For this review, take the finished solid that the model builds, in its own axes (mm). Face numbers are marked on the shaded views. A direction names the side the tool comes from. Give positions to 0.01 mm unless a question says otherwise; leave off trailing zeros. Loops run counter-clockwise (first coordinate to the right, second up) from the corner with the lowest first, then second, coordinate; pieces in that order, holes last. Notation, with made-up numbers: (40, 59.25) - (70, 59.25) arc R31 ccw to (70, 93.25) - close; hole circle Ø10 at (77.5, -6.5). An arc over 180 degrees is marked (long way). Use CSV: the item, a comma, the result in double quotes. Start each with the question number.
1. Take a section at B-B on z = 17.5. Give the boundary of the cut face in (x, y).
2. Wall thickness on line 1 (X direction, y = -42, z = 8.5); line 2 (X direction, y = 23.5, z = 22.5); line 3 (X direction, y = 40, z = -0.5): over which ranges is each line inside the solid? List them lowest first.
3. Take a section at C-C on y = -20.5. Give the boundary of the cut face in (x, z).
4. For the marked faces 1 and 2, list the 3-axis set-ups (+Z, -Z, +X, -X, +Y, -Y) from which the entire face can be reached by the end or side of a thin tool; tool diameter is ignored.
5. For pin 1 (5.5 mm diameter, centred on x = 12.96, y = -44.14, fed in from +Z); pin 2 (10 mm diameter, centred on x = -29.54, y = 5.21, fed in from +Z); pin 3 (7 mm diameter, centred on x = 77.94, y = -43.87, fed in from -Z); pin 4 (5 mm diameter, centred on y = 69.5, z = -5, fed in from +X), all flat-tipped, find the tip position at first contact; note any pin that passes through.
6. Take a section at A-A on y = 30. Give the boundary of the cut face in (x, z), plus the area to 3 significant figures.
7. Mouldability with a two-part tool opening along Y and no side actions: class the marked faces 3, 4 and 5 as pulls with the +Y half, pulls with the -Y half, needs draft (parallel to the pull), parting line crosses it, or undercut.
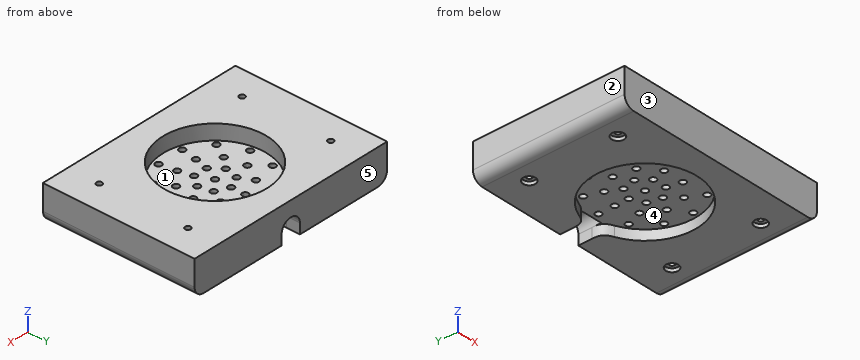
```python
from build123d import *

# Parameters (mm, degrees)
SKETCH1_R                                 = 56
BOSS_EXTRUDE1_DEPTH                       = 25
SKETCH2_W                                 = 210
SKETCH2_H                                 = 150
SKETCH2_R                                 = 51.5
BOSS_EXTRUDE2_DEPTH                       = 35
SKETCH3_R                                 = 3.1
CUT_EXTRUDE1_DEPTH                        = 132.434394281
SKETCH7_R                                 = 51.5
CUT_EXTRUDE2_DEPTH                        = 15
CBORE_FOR_M5_HEX_BOLT_GRADE_C1_AT_2_COUNT = 2
CBORE_FOR_M5_HEX_BOLT_GRADE_C1_AT_2_PITCH = 87.749643874
CBORE_FOR_M5_HEX_BOLT_GRADE_C1_AT_3_COUNT = 2
CBORE_FOR_M5_HEX_BOLT_GRADE_C1_AT_3_PITCH = 155.884572681
CBORE_FOR_M5_HEX_BOLT_GRADE_C1_AT_4_COUNT = 2
CBORE_FOR_M5_HEX_BOLT_GRADE_C1_AT_4_PITCH = 178.8854382
SKETCH17_W                                = 20
SKETCH17_H                                = 40
CUT_EXTRUDE4_DEPTH                        = 10
SKETCH18_R                                = 10
CUT_EXTRUDE5_DEPTH                        = 22.5
FILLET6_R                                 = 10


with BuildPart() as part:
    # Sketch1 → Boss-Extrude1 (new body)
    with BuildSketch(Plane.XY):
        Circle(SKETCH1_R)
    extrude(amount=BOSS_EXTRUDE1_DEPTH)

    # Sketch2 → Boss-Extrude2 (add)
    with BuildSketch(Plane.XY.offset(25)):
        Rectangle(SKETCH2_W, SKETCH2_H)
        Circle(SKETCH2_R, mode=Mode.SUBTRACT)
    extrude(amount=-BOSS_EXTRUDE2_DEPTH)

    # Sketch3 → Cut-Extrude1 (cut, through all)
    with BuildSketch(Plane(origin=(0, 0, 0), x_dir=(-1, 0, 0), z_dir=(0, 0, -1))):
        with Locations((0, 46)):
            Circle(SKETCH3_R)
        with Locations((0, 30)):
            Circle(SKETCH3_R)
        with Locations((0, 16)):
            Circle(SKETCH3_R)
        with Locations((12.509303719, 9.97583683)):
            Circle(SKETCH3_R)
        with Locations((15.598846595, -3.560334943)):
            Circle(SKETCH3_R)
        with Locations((6.942139826, -14.415501886)):
            Circle(SKETCH3_R)
        with Locations((-6.942139826, -14.415501886)):
            Circle(SKETCH3_R)
        with Locations((-15.598846595, -3.560334943)):
            Circle(SKETCH3_R)
        with Locations((-12.509303719, 9.97583683)):
            Circle(SKETCH3_R)
        with Locations((19.283628291, 22.981333294)):
            Circle(SKETCH3_R)
        with Locations((29.54423259, 5.20944533)):
            Circle(SKETCH3_R)
        with Locations((25.980762114, -15)):
            Circle(SKETCH3_R)
        with Locations((10.2606043, -28.190778624)):
            Circle(SKETCH3_R)
        with Locations((-10.2606043, -28.190778624)):
            Circle(SKETCH3_R)
        with Locations((-25.980762114, -15)):
            Circle(SKETCH3_R)
        with Locations((-29.54423259, 5.20944533)):
            Circle(SKETCH3_R)
        with Locations((-19.283628291, 22.981333294)):
            Circle(SKETCH3_R)
        with Locations((24.869477603, 38.69766251)):
            Circle(SKETCH3_R)
        with Locations((41.843071786, 19.109090598)):
            Circle(SKETCH3_R)
        with Locations((45.531786327, -6.546482561)):
            Circle(SKETCH3_R)
        with Locations((34.76448042, -30.123593761)):
            Circle(SKETCH3_R)
        with Locations((12.959697615, -44.136676786)):
            Circle(SKETCH3_R)
        with Locations((-12.959697615, -44.136676786)):
            Circle(SKETCH3_R)
        with Locations((-34.76448042, -30.123593761)):
            Circle(SKETCH3_R)
        with Locations((-45.531786327, -6.546482561)):
            Circle(SKETCH3_R)
        with Locations((-41.843071786, 19.109090598)):
            Circle(SKETCH3_R)
        with Locations((-24.869477603, 38.69766251)):
            Circle(SKETCH3_R)
        Circle(SKETCH3_R)
    extrude(amount=-CUT_EXTRUDE1_DEPTH, mode=Mode.SUBTRACT)

    # Sketch7 → Cut-Extrude2 (cut)
    with BuildSketch(Plane.XY.offset(25)):
        Circle(SKETCH7_R)
    extrude(amount=-CUT_EXTRUDE2_DEPTH, mode=Mode.SUBTRACT)

    # Sketch12 → CBORE for M5 Hex Bolt Grade C1 (revolve, cut)
    with BuildSketch(Plane(origin=(77.942286341, 43.874821937, -10), x_dir=(0, 1, 0), z_dir=(1, 0, 0))):
        Polygon((0, 0), (0, 35), (2.75, 35), (2.75, 3.5), (6.119, 3.5), (6.119, 0.024142219), (6.144, 0), align=None)
    cbore_for_m5_hex_bolt_grade_c1 = revolve(axis=Axis((77.942286341, 43.874821937, -16.35), (0, 0, 1)), mode=Mode.SUBTRACT)

    # CBORE for M5 Hex Bolt Grade C1 at 2: CBORE for M5 Hex Bolt Grade C1 ×2
    with Locations(*[(0, -i * CBORE_FOR_M5_HEX_BOLT_GRADE_C1_AT_2_PITCH, 0) for i in range(1, CBORE_FOR_M5_HEX_BOLT_GRADE_C1_AT_2_COUNT)]):
        add(cbore_for_m5_hex_bolt_grade_c1, mode=Mode.SUBTRACT)

    # CBORE for M5 Hex Bolt Grade C1 at 3: CBORE for M5 Hex Bolt Grade C1 ×2
    with Locations(*[(-i * CBORE_FOR_M5_HEX_BOLT_GRADE_C1_AT_3_PITCH, 0, 0) for i in range(1, CBORE_FOR_M5_HEX_BOLT_GRADE_C1_AT_3_COUNT)]):
        add(cbore_for_m5_hex_bolt_grade_c1, mode=Mode.SUBTRACT)

    # CBORE for M5 Hex Bolt Grade C1 at 4: CBORE for M5 Hex Bolt Grade C1 ×2
    with Locations(*[Vector(-0.8714212528966683, -0.4905354217587157, 0) * (i * CBORE_FOR_M5_HEX_BOLT_GRADE_C1_AT_4_PITCH) for i in range(1, CBORE_FOR_M5_HEX_BOLT_GRADE_C1_AT_4_COUNT)]):
        add(cbore_for_m5_hex_bolt_grade_c1, mode=Mode.SUBTRACT)

    # Sketch17 → Cut-Extrude4 (cut)
    with BuildSketch(Plane(origin=(0, 0, -10), x_dir=(-1, 0, 0), z_dir=(0, 0, -1))):
        with Locations((0, 65.672027366)):
            Rectangle(SKETCH17_W, SKETCH17_H)
    extrude(amount=-CUT_EXTRUDE4_DEPTH, mode=Mode.SUBTRACT)

    # Sketch18 → Cut-Extrude5 (cut)
    with BuildSketch(Plane(origin=(0, 75, 0), x_dir=(1, 0, 0), z_dir=(0, 1, 0))):
        Circle(SKETCH18_R)
    extrude(amount=-CUT_EXTRUDE5_DEPTH, mode=Mode.SUBTRACT)

    # Fillet6
    fillet6_edges = [part.edges().sort_by_distance(p)[0] for p in [
        (-105, 0, -10),
        (105, 0, -10),
    ]]
    fillet(fillet6_edges, radius=FILLET6_R)

    # Fillet7
    # a fillet whose section is not a circle: 15 mm, written as the material it takes off along each edge
    with BuildSketch(Plane(origin=(10, 50.519798099, -37.75508112), x_dir=(0, 1, 0), z_dir=(0, 0, 1))) as fillet7_piece_1:
        with BuildLine():
            Bezier((11.102032448, 0), (1.000093014, 0), (-2.797628578, -9.360902256), weights=[1, 1.5, 1])
            ThreePointArc((-2.797628578, -9.360902256), (-1.176331731, -4.746942962), (0, 0))
            Line((0, 0), (11.102032448, 0))
        make_face()
    extrude(amount=37.75508112, mode=Mode.SUBTRACT)
    with BuildSketch(Plane(origin=(-10, 50.519798099, -37.75508112), x_dir=(0, 1, 0), z_dir=(0, 0, 1))) as fillet7_piece_2:
        with BuildLine():
            Bezier((11.102032448, 0), (1.000093014, 0), (-2.797628578, 9.360902256), weights=[1, 1.5, 1])
            ThreePointArc((-2.797628578, 9.360902256), (-1.176331731, 4.746942962), (0, 0))
            Line((0, 0), (11.102032448, 0))
        make_face()
    extrude(amount=37.75508112, mode=Mode.SUBTRACT)


solid = part.part
```
Check result:
1,outline,"(-105, -75) - (105, -75) - (105, 75) - (-105, 75) - close; hole circle Ø5.5 at (-77.94, -43.87); hole circle Ø5.5 at (-77.94, 43.87); hole circle Ø103 at (0, 0); hole circle Ø5.5 at (77.94, -43.87); hole circle Ø5.5 at (77.94, 43.87)"
2,line 1,"x = -105 to -79.95, -75.93 to -15.21, -10.71 to 10.71, 15.21 to 75.93, 79.95 to 105"
2,line 2,"x = -105 to -45.83, 45.83 to 105"
2,line 3,"x = -104.99 to -32.44, 32.44 to 104.99"
3,outline,"(-105, 0) arc R10 ccw to (-95, -10) - (-47.24, -10) - (-47.24, 0) - (47.24, 0) - (47.24, -10) - (95, -10) arc R10 ccw to (105, 0) - (105, 25) - (47.24, 25) - (47.24, 10) - (-47.24, 10) - (-47.24, 25) - (-105, 25) - close"
4,face 1,"+Z"
4,face 2,"+Z, -Z, -X, +Y, -Y"
5,pin 1,"passes through"
5,pin 2,"stops at z = 10"
5,pin 3,"stops at z = -6.5"
5,pin 4,"stops at x = 104.68"
6,outline,"(-105, 0) arc R10 ccw to (-95, -10) - (-41.86, -10) - (-41.86, 0) - (-3.1, 0) - (-3.1, 10) - (-41.86, 10) - (-41.86, 25) - (-105, 25) - close; (3.1, 0) - (41.86, 0) - (41.86, -10) - (95, -10) arc R10 ccw to (105, 0) - (105, 25) - (41.86, 25) - (41.86, 10) - (3.1, 10) - close"
6,area,"5,150 mm²"
7,face 3,"pulls with the -Y half"
7,face 4,"undercut"
7,face 5,"pulls with the +Y half"
